Autodesk Inventor part; units mm, degrees
ref_plane "YZ Plane" through (0, 0, 0) normal (1, 0, 0) x (0, 1, 0)
ref_plane "XY Plane" through (0, 0, 0) normal (0, 0, 1) x (1, 0, 0)
ref_plane "工作平面1" through (0, 0, 1.5) normal (0, 0, 1) x (1, 0, 0)
sketch "草圖1" plane through (0, 0, 0) normal (0, 0, 1) x (1, 0, 0)
  line L0 (0, 6) -> (0, -6)
  line L1 (0, -6) -> (-139, -6)
  line L2 (-139, -6) -> (-139, 6)
  line L3 (-148, 2) -> (-139, 2)
  line L4 (-139, 2) -> (-139, -2)
  line L5 (-139, -2) -> (-148, -2)
  line L6 (-148, -2) -> (-148, 2)
  line L7 (-207.2, 0) -> (207.2, 0)
  line L8 (0, -9.6) -> (0, 15.6)
  line L9 (0, -6) -> (139, -6)
  line L10 (139, -6) -> (139, 6)
  line L11 (148, 2) -> (139, 2)
  line L12 (139, -2) -> (148, -2)
  line L13 (148, -2) -> (148, 2)
  line L14 (-148, -2) -> (-139, -2)
  line L15 (-139, -2) -> (-139, -6)
  line L16 (139, -6) -> (139, -2)
  line L17 (139, -2) -> (148, -2)
  line L18 (148, -2) -> (148, 2)
  line L19 (148, 2) -> (139, 2)
  line L20 (139, 2) -> (139, 6)
  line L21 (-139, 6) -> (-139, 2)
  line L22 (-139, 2) -> (-148, 2)
  line L23 (-148, 2) -> (-148, -2)
  line L24 (-97.5, 7) -> (-97.5, 12)
  line L25 (-97.5, 12) -> (-87.5, 12)
  line L26 (-90, 7) -> (-97.5, 7)
  line L27 (-90, 7) -> (-90, 5)
  line L28 (-90, 5) -> (-91, 5)
  line L29 (-91, 5) -> (-91, 6)
  line L30 (97.5, 7) -> (97.5, 12)
  line L31 (97.5, 12) -> (87.5, 12)
  line L32 (90, 7) -> (97.5, 7)
  line L33 (90, 7) -> (90, 5)
  line L34 (90, 5) -> (91, 5)
  line L35 (91, 5) -> (91, 6)
  line L36 (-139, 6) -> (-91, 6)
  line L37 (-85.5, 6) -> (85.5, 6)
  line L38 (91, 6) -> (139, 6)
  line L39 (-87.5, 12) -> (-85.5, 12)
  line L40 (-85.5, 12) -> (-85.5, 6)
  line L41 (87.5, 12) -> (85.5, 12)
  line L42 (85.5, 12) -> (85.5, 6)
  point P0 (0, 0)
  point P1 (-139, 2)
  dimension "d2" = 4
  dimension "d13" = 2
  dimension "d14" = 2
  dimension "d17" = 12
extrude "擠出1" add sketch "草圖1" along normal blind 3
ref_plane "工作平面1" through (0, 0, 1.5) normal (0, 0, 1) x (1, 0, 0)
sketch "草圖7" plane through (0, 0, 3) normal (0, 0, 1) x (1, 0, 0)
  line L0 (0, 1.45) -> (-139, 1.45)
  line L1 (-139, 1.45) -> (-139, -1.45)
  line L2 (-139, -1.45) -> (0, -1.45)
  line L3 (0, -1.45) -> (0, 1.45)
  line L4 (91, 6) -> (91, 5)
  line L5 (91, 5) -> (90, 5)
  line L6 (90, 5) -> (90, 7)
  line L7 (90, 7) -> (97.5, 7)
  line L8 (97.5, 7) -> (97.5, 12)
  line L9 (97.5, 12) -> (85.5, 12)
  line L10 (85.5, 12) -> (85.5, 6)
  line L11 (85.5, 6) -> (-85.5, 6)
  line L12 (-85.5, 6) -> (-85.5, 12)
  line L13 (-85.5, 12) -> (-97.5, 12)
  line L14 (-97.5, 12) -> (-97.5, 7)
  line L15 (-97.5, 7) -> (-90, 7)
  line L16 (-90, 7) -> (-90, 5)
  line L17 (-90, 5) -> (-91, 5)
  line L18 (-91, 5) -> (-91, 6)
  line L19 (-91, 6) -> (-139, 6)
  line L20 (-139, 6) -> (-139, 2)
  line L21 (-139, 2) -> (-148, 2)
  line L22 (-148, 2) -> (-148, -2)
  line L23 (-148, -2) -> (-139, -2)
  line L24 (-139, -2) -> (-139, -6)
  line L25 (-139, -6) -> (139, -6)
  line L26 (139, -6) -> (139, -2)
  line L27 (139, -2) -> (148, -2)
  line L28 (148, -2) -> (148, 2)
  line L29 (148, 2) -> (139, 2)
  line L30 (139, 2) -> (139, 6)
  line L31 (139, 6) -> (91, 6)
  line L32 (-139, 1.45) -> (-139, 2)
  line L33 (-148, -2) -> (-139, -2)
  line L34 (-139, -1.45) -> (-139, -2)
  point P0 (0, 0)
  point P1 (0, 0)
  dimension "d39" = 139
  dimension "d40" = 2.9
extrude "擠出5" cut sketch "草圖7" against normal up to surface (3 mm away) contours L3 L2 L1 L0 | L1 L34 L23 L22 L21 L32
properties part number "rod_6"
Can you work these out from the model? Positions are in its coordinate system, mm. Round coordinates to 2 decimals unless told otherwise and drop trailing zeros. Loops run counter-clockwise (first coordinate to the right, second up) from the corner with the lowest first, then second, coordinate; pieces in that order, holes last. Notation, with made-up numbers: (48, 44) - (95, 44) arc R20 ccw to (95, 70) - close; hole circle Ø10 at (41, 3.25). An arc over 180 degrees is marked (long way). Write item = value, one per line. Start each with the question number.
(1) If I drill on probe 1 along Y at (x, z) = (-41, 0.2); probe 2 along X at (y, z) = (9.75, 2.65); probe 3 along Y at (x, z) = (121.5, 0.25), over which ranges is the centre line in solid material (lowest first)? Write a range as [from, to].
(2) For P1, Ø1.5, axis at x = -18.5, z = 1, coming from the +Y side; P2, Ø0.9, axis at x = 144.5, z = 1.5, coming from the +Y side; P3, Ø0.8, axis at y = 5.5, z = 1.5, coming from the +X side, each with a flat end and sliding along its axis, tell me the tip position at first contact or that it passes through.
(3) If we section it at C-C (x = 18): Please give me the cut outline in (y, z), and give its area (3 significant figures).
(4) If we section it at A-A (x = -35.5): Please give me the cut outline in (y, z).
(5) If we section it at B-B (z = 2.55): Please give me the cut outline in (x, y), and give its area (3 significant figures).
Ans:
q1.probe_1 = [-6, -1.45], [1.45, 6]
q1.probe_2 = [-97.5, -85.5], [85.5, 97.5]
q1.probe_3 = [-6, 6]
q2.P1 = 6
q2.P2 = 2
q2.P3 = 139
q3.outline = (-6, 0) - (6, 0) - (6, 3) - (-6, 3) - close
q3.area = 36.0 mm²
q4.outline = (-6, 0) - (-1.45, 0) - (-1.45, 3) - (-6, 3) - close; (1.45, 0) - (6, 0) - (6, 3) - (1.45, 3) - close
q5.outline = (-139, -6) - (139, -6) - (139, -2) - (148, -2) - (148, 2) - (139, 2) - (139, 6) - (91, 6) - (91, 5) - (90, 5) - (90, 7) - (97.5, 7) - (97.5, 12) - (85.5, 12) - (85.5, 6) - (-85.5, 6) - (-85.5, 12) - (-97.5, 12) - (-97.5, 7) - (-90, 7) - (-90, 5) - (-91, 5) - (-91, 6) - (-139, 6) - (-139, 1.45) - (0, 1.45) - (0, -1.45) - (-139, -1.45) - close
q5.area = 3,100 mm²
